from build123d import *

# Parameters (mm, degrees)
BOX_W           = 30
BOX_H           = 30
BOX_DEPTH       = 30
SKETCH_R        = 3.5
POCKET_DEPTH    = 30.001
SKETCH004_R     = 7
POCKET001_DEPTH = 13
SKETCH001_R     = 7
POCKET002_DEPTH = 13
SKETCH003_R     = 12.5
POCKET003_DEPTH = 30.001
SKETCH002_R     = 12.5
POCKET004_DEPTH = 30.001


with BuildPart() as part:
    # Box → Box (new body)
    with BuildSketch(Plane.XY):
        with Locations((15, 15)):
            Rectangle(BOX_W, BOX_H)
    extrude(amount=BOX_DEPTH)

    # Sketch → Pocket (cut, through all)
    with BuildSketch(Plane.XY.offset(30)):
        with Locations((15, 15)):
            Circle(SKETCH_R)
    extrude(amount=-POCKET_DEPTH, mode=Mode.SUBTRACT)

    # Sketch004 → Pocket001 (cut)
    with BuildSketch(Plane.XY.offset(30)):
        with Locations((15, 15)):
            Circle(SKETCH004_R)
    extrude(amount=-POCKET001_DEPTH, mode=Mode.SUBTRACT)

    # Sketch001 → Pocket002 (cut)
    with BuildSketch(Plane(origin=(0, 0, 0), x_dir=(1, 0, 0), z_dir=(0, 0, -1))):
        with Locations((15, -15)):
            Circle(SKETCH001_R)
    extrude(amount=-POCKET002_DEPTH, mode=Mode.SUBTRACT)

    # Sketch003 → Pocket003 (cut, through all)
    with BuildSketch(Plane(origin=(0, 0, 0), x_dir=(0, -1, 0), z_dir=(-1, 0, 0))):
        with Locations((-15, 30)):
            Circle(SKETCH003_R)
    extrude(amount=-POCKET003_DEPTH, mode=Mode.SUBTRACT)

    # Sketch002 → Pocket004 (cut, through all)
    with BuildSketch(Plane.XZ):
        with Locations((15, 0)):
            Circle(SKETCH002_R)
    extrude(amount=-POCKET004_DEPTH, mode=Mode.SUBTRACT)


solid = part.part
The model under review builds one solid part; all positions refer to its coordinate system, in mm. A direction names the side the tool comes from. Give positions to 0.01 mm unless a question says otherwise; leave off trailing zeros. Loops run counter-clockwise (first coordinate to the right, second up) from the corner with the lowest first, then second, coordinate; pieces in that order, holes last. Notation, with made-up numbers: (15, 86.25) -> (60, 86.25) arc R26 cw to (60, 118.25) -> close; hole circle Ø6 at (22, -36). An arc over 180 degrees is marked (long way). Answer as a JSON object with one key per item and string values. Group by question number.
Q1. Draft analysis for pull direction X (two halves, no side actions). For faces 1 (the flat face through (0, 15, 11)), 2 (the cylindrical face through (9.84, 19.73, 18.05)), 3 (the flat face through (1, 15, 0)), state which applies: pulls with the +X half, pulls with the -X half, needs draft (parallel to the pull), parting line crosses it, or undercut.
Q2. Take a section at A-A (x = 15). Write out the cut boundary in (y, z), plus the area to 3 significant figures.
Q3. Wall thickness on line 1 along Y through (x, z) = (15, 14); line 2 along Y through (x, z) = (15, 18.85); line 3 along Z through (x, y) = (17, 12): over which ranges is each line inside the solid? List them lowest first.
Q4. Take a section at C-C (z = 19). Write out the cut boundary in (x, y), plus the area to 3 significant figures.
Q5. Insertion check: pin 1 (3 mm diameter, centred on x = 19.5, y = 16, fed in from -Z); pin 2 (18 mm diameter, centred on x = 15, y = 15, fed in from +Z); pin 3 (8 mm diameter, centred on x = 15, y = 15, fed in from +Z). Each pin has a flat end and moves straight along its axis. Give the tip position at first contact, or say it passes through.
Q6. Take a section at D-D (x = 27). Write out the cut boundary in (y, z), plus the area to 3 significant figures.
Q7. Take a section at B-B (y = 15). Write out the cut boundary in (x, z).
Q8. Tool access review of faces 4 (the flat face through (18, 12, 17)), 5 (the flat face through (29, 15, 0)), 6 (the flat face through (18, 18, 13)): name each direction out of +Z, -Z, +X, -X, +Y, -Y from which nothing blocks a thin tool from reaching the whole face with its end or side.
Answer below:
{
 "1": {"face 1": "pulls with the -X half", "face 2": "undercut", "face 3": "needs draft"},
 "2": {"outline": "(0, 12.5) -> (8, 12.5) -> (8, 13) -> (11.5, 13) -> (11.5, 17) -> (8, 17) -> (8, 19.64) arc R12.5 cw to (2.5, 30) -> (0, 30) -> close; (18.5, 13) -> (22, 13) -> (22, 12.5) -> (30, 12.5) -> (30, 30) -> (27.5, 30) arc R12.5 cw to (22, 19.64) -> (22, 17) -> (18.5, 17) -> close", "area": "228 mm2"},
 "3": {"line 1": "y = 0 to 11.5, 18.5 to 30", "line 2": "y = 0 to 8, 22 to 30", "line 3": "z = 13 to 17"},
 "4": {"outline": "(0, 0) -> (30, 0) -> (30, 9.06) -> (18.71, 9.06) arc R7 cw to (11.29, 9.06) -> (0, 9.06) -> close; (0, 20.94) -> (11.29, 20.94) arc R7 cw to (18.71, 20.94) -> (30, 20.94) -> (30, 30) -> (0, 30) -> close", "area": "533 mm2"},
 "5": {"pin 1": "stops at z = 13", "pin 2": "stops at z = 21.33", "pin 3": "stops at z = 17"},
 "6": {"outline": "(0, 3.5) -> (30, 3.5) -> (30, 30) -> (27.5, 30) arc R12.5 cw to (2.5, 30) -> (0, 30) -> close", "area": "550 mm2"},
 "7": {"outline": "(0, 0) -> (2.5, 0) arc R12.5 cw to (8, 10.36) -> (8, 13) -> (11.5, 13) -> (11.5, 17) -> (8, 17) -> (8, 17.5) -> (0, 17.5) -> close; (18.5, 13) -> (22, 13) -> (22, 10.36) arc R12.5 cw to (27.5, 0) -> (30, 0) -> (30, 17.5) -> (22, 17.5) -> (22, 17) -> (18.5, 17) -> close"},
 "8": {"face 4": "+Z", "face 5": "-Z, +X, -X, +Y, -Y", "face 6": "-Z"}
}
